The figure shows three views and two pictorial views of one solid part (mm, origin at its lowest corner). Answer the questions. A direction names the side the tool comes from. Give positions to 0.01 mm unless a question says otherwise; leave off trailing zeros. Loops run counter-clockwise (first coordinate to the right, second up) from the corner with the lowest first, then second, coordinate; pieces in that order, holes last. Notation, with made-up numbers: (45, -30.5) - (63, -30.5) arc R18 ccw to (63, -4.5) - close; hole circle Ø11 at (85, 41.5). An arc over 180 degrees is marked (long way). Use CSV: the item, a comma, the result in double quotes.
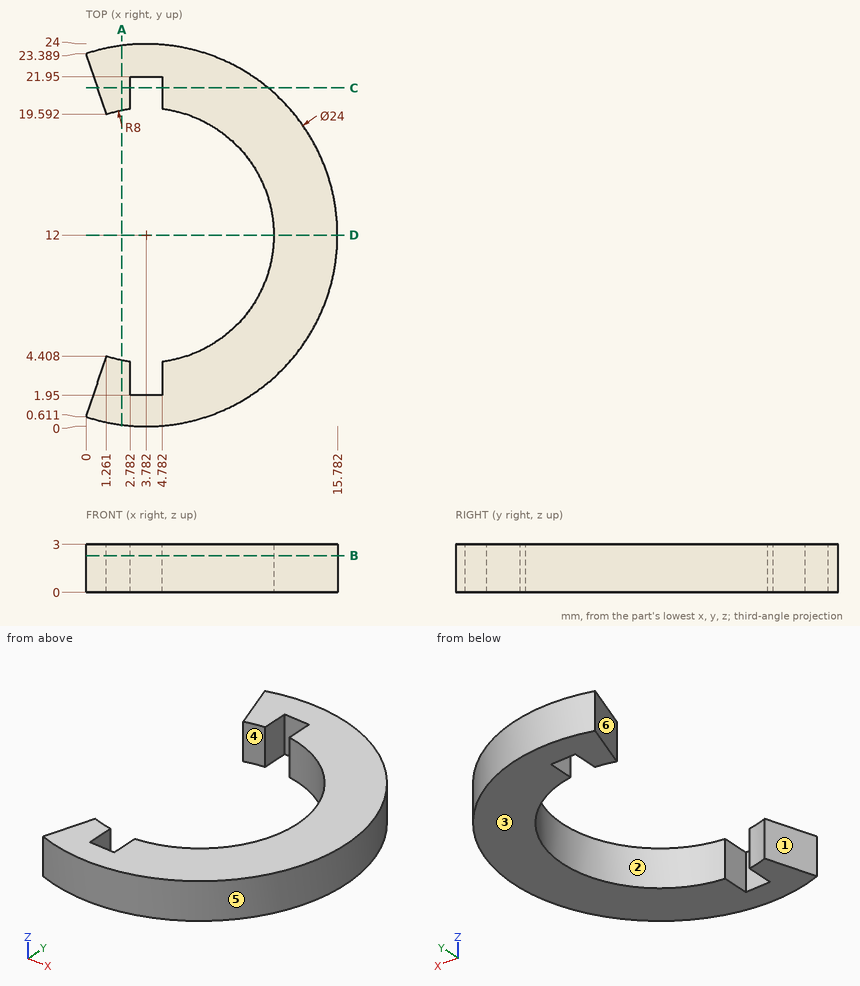
Item 1: Find the intervals of material crossed by line 1 (Y direction, x = 3.5, z = 0.55); line 2 (X direction, y = 12, z = 1.7); line 3 (Y direction, x = 10, z = 2.35) (1 decimal), in increasing order.
Determined:
line 1,"y = 0 to 1.95, 21.95 to 24"
line 2,"x = 11.78 to 15.78"
line 3,"y = 1.7 to 7, 17 to 22.3"
Item 2: A cutting plane is placed at D-D on y = 12. Determine the outline of the cut face in (x, z), and give its area (3 significant figures).
Determined:
outline,"(11.78, 0) - (15.78, 0) - (15.78, 3) - (11.78, 3) - close"
area,"12.0 mm²"
Item 3: A cutting plane is placed at C-C on y = 21.25. Determine the outline of the cut face in (x, z).
Determined:
outline,"(0.71, 0) - (2.78, 0) - (2.78, 3) - (0.71, 3) - close; (4.78, 0) - (11.43, 0) - (11.43, 3) - (4.78, 3) - close"
Item 4: Given P1, Ø0.6, axis at y = 3, z = 1, coming from the -X side; P2, Ø1, axis at y = 21, z = 2, coming from the +X side; P3, Ø1.1, axis at y = 3.5, z = 2, coming from the +X side, each flat-ended and moving along its own axis, determine where each tip first touches the part or whether it passes through.
Determined:
P1,"stops at x = 0.69"
P2,"stops at x = 12.25"
P3,"stops at x = 12.77"
Item 5: The mould has two halves that part along X. Classify the marked faces 4, 5 and 6: pulls with the +X half, pulls with the -X half, needs draft (parallel to the pull), parting line crosses it, or undercut.
Determined:
face 4,"undercut"
face 5,"parting line crosses it"
face 6,"pulls with the -X half"
Item 6: A cutting plane is placed at B-B on z = 2.3. Determine the outline of the cut face in (x, y), and give its area (3 significant figures).
Determined:
outline,"(0, 0.61) arc R12 ccw (long way) to (0, 23.39) - (1.26, 19.59) arc R8 cw to (2.78, 19.94) - (2.78, 21.95) - (4.78, 21.95) - (4.78, 19.94) arc R8 cw to (4.78, 4.06) - (4.78, 1.95) - (2.78, 1.95) - (2.78, 4.06) arc R8 cw to (1.26, 4.41) - close"
area,"143 mm²"
Item 7: For the marked faces 1, 2 and 3, determine the directions among +Z, -Z, +X, -X, +Y, -Y from which every point of the face is accessible in a straight line to the end or side of a thin tool.
Determined:
face 1,"+Z, -Z, -X"
face 2,"+Z, -Z"
face 3,"-Z, +X, -X, +Y, -Y"
Item 8: A cutting plane is placed at A-A on x = 2.25. Determine the outline of the cut face in (y, z).
Determined:
outline,"(0.1, 0) - (4.15, 0) - (4.15, 3) - (0.1, 3) - close; (19.85, 0) - (23.9, 0) - (23.9, 3) - (19.85, 3) - close"
